from build123d import *

# Parameters (mm, degrees)
PAD_DEPTH            = 60
SKETCH001_R          = 1.45
POCKET_DEPTH         = 59
SKETCH002_R          = 1.5
POCKET001_DEPTH      = 13.501
POCKET001_DEPTH_BACK = -73.501
SKETCH003_R          = 7.75
POCKET002_DEPTH      = 333.774629
POLARPATTERN_COUNT   = 4
CHAMFER_SIZE         = 2


with BuildPart() as part:
    # Sketch → Pad (new body)
    with BuildSketch(Plane.XY):
        with BuildLine():
            Line((-39.5, 43.5), (39.5, 43.5))
            ThreePointArc((43.5, 39.5), (42.328427, 42.328427), (39.5, 43.5))
            Line((43.5, 39.5), (43.5, -39.5))
            ThreePointArc((39.5, -43.5), (42.328427, -42.328427), (43.5, -39.5))
            Line((39.5, -43.5), (-39.5, -43.5))
            ThreePointArc((-43.5, -39.5), (-42.328427, -42.328427), (-39.5, -43.5))
            Line((-43.5, -39.5), (-43.5, 39.5))
            ThreePointArc((-39.5, 43.5), (-42.328427, 42.328427), (-43.5, 39.5))
        make_face()
    extrude(amount=PAD_DEPTH)

    # Sketch001 (on Face10 of Pad) → Pocket (cut)
    with BuildSketch(Plane.XY.offset(60)):
        with Locations((-33, 33)):
            Circle(SKETCH001_R)
        with Locations((33, 33)):
            Circle(SKETCH001_R)
        with Locations((33, -33)):
            Circle(SKETCH001_R)
        with Locations((-33, -33)):
            Circle(SKETCH001_R)
        with BuildLine():
            Line((-30, 33), (-30, 41))
            Line((-30, 41), (30, 41))
            Line((30, 41), (30, 33))
            ThreePointArc((30, 33), (30.87868, 30.87868), (33, 30))
            Line((33, 30), (41, 30))
            Line((41, 30), (41, -30))
            Line((41, -30), (33, -30))
            ThreePointArc((33, -30), (30.87868, -30.87868), (30, -33))
            Line((30, -33), (30, -41))
            Line((30, -41), (-30, -41))
            Line((-30, -41), (-30, -33))
            ThreePointArc((-30, -33), (-30.87868, -30.87868), (-33, -30))
            Line((-33, -30), (-41, -30))
            Line((-41, -30), (-41, 30))
            Line((-41, 30), (-33, 30))
            ThreePointArc((-33, 30), (-30.87868, 30.87868), (-30, 33))
        make_face()
    extrude(amount=-POCKET_DEPTH, mode=Mode.SUBTRACT)

    # Sketch002 (on Face26 of Pocket) → Pocket001 (cut, two sides)
    with BuildSketch(Plane.XZ.offset(-30)) as pocket001_sk:
        with Locations((-37, 55)):
            Circle(SKETCH002_R)
        with Locations((37, 55)):
            Circle(SKETCH002_R)
        with Locations((-37, 6)):
            Circle(SKETCH002_R)
        with Locations((37, 6)):
            Circle(SKETCH002_R)
    extrude(amount=-POCKET001_DEPTH, mode=Mode.SUBTRACT)
    extrude(pocket001_sk.sketch, amount=-POCKET001_DEPTH_BACK, mode=Mode.SUBTRACT)

    # Sketch003 → Pocket002 (cut, through all)
    with BuildSketch(Plane.XY):
        with Locations((20, 20)):
            Circle(SKETCH003_R)
    pocket002 = extrude(amount=POCKET002_DEPTH, mode=Mode.SUBTRACT)

    # PolarPattern: Pocket002 ×4 about axis
    polarpattern_axis = Axis((0, 0, 0), (0, 0, 1))
    for i in range(1, POLARPATTERN_COUNT):
        add(pocket002.rotate(polarpattern_axis, i * 360 / POLARPATTERN_COUNT), mode=Mode.SUBTRACT)

    # Chamfer
    chamfer_edges = [part.edges().sort_by_distance(p)[0] for p in [
        (-37, 30, 1),
        (0, 41, 1),
        (30, 37, 1),
        (-41, 0, 1),
        (-30, -37, 1),
        (0, -41, 1),
        (41, 0, 1),
        (37, -30, 1),
    ]]
    chamfer(chamfer_edges, length=CHAMFER_SIZE)


solid = part.part
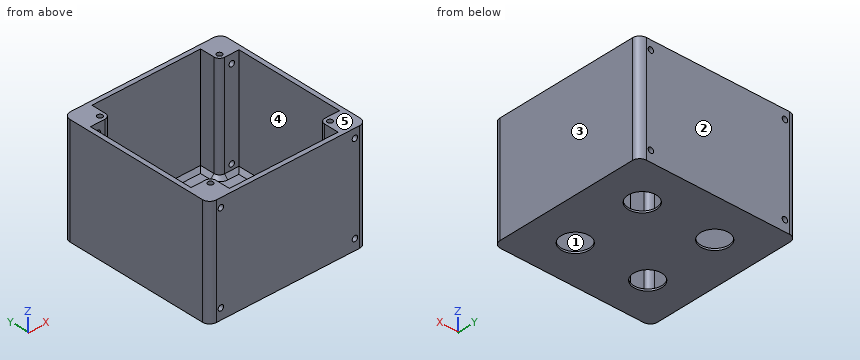
Part model, mm, in its own coordinate system. Face numbers are marked on the shaded views. A direction names the side the tool comes from. Give positions to 0.01 mm unless a question says otherwise; leave off trailing zeros. Write each loop counter-clockwise with the first axis right and the second up, starting at its lowest first coordinate (ties: lowest second). Pieces come first, ordered by that corner, then holes.
1) Probe L1, parallel to Z at x = 37, y = 37; L2, parallel to X at y = -37, z = 55; L3, parallel to Y at x = 20, z = 0.65. List the from-to ranges inside material, lowest first.
Resolved:
L1: z = 0 to 4.5, 7.5 to 53.5, 56.5 to 60
L2: x = -43.5 to -38.5, -35.5 to -30, 30 to 35.5, 38.5 to 43.5
L3: y = -43.5 to -27.75, -12.25 to 12.25, 27.75 to 43.5
2) Which spindle directions (+Z, -Z, +X, -X, +Y, -Y) get a long thin tool onto all of the face, cutting with end or side? Do the marked faces 4 and 5. Say none if no direction does.
Resolved:
face 4: +Z
face 5: +Z, +X, -X, +Y, -Y
3) Two-plate mould, pull along Y, no slides. Class the marked faces 1, 2 and 3: released by +Y, released by -Y, zero draft, split by the parting line, or undercut.
Resolved:
face 1: undercut
face 2: released by +Y
face 3: zero draft
4) Cut at C-C on z = 48. Write the cut outline in (x, y), then the cut area to 3 significant figures.
Resolved:
outline: (-43.5, -39.5) arc R4 ccw to (-39.5, -43.5) - (39.5, -43.5) arc R4 ccw to (43.5, -39.5) - (43.5, 39.5) arc R4 ccw to (39.5, 43.5) - (-39.5, 43.5) arc R4 ccw to (-43.5, 39.5) - close; hole (-41, -30) - (-33, -30) arc R3 cw to (-30, -33) - (-30, -41) - (30, -41) - (30, -33) arc R3 cw to (33, -30) - (41, -30) - (41, 30) - (33, 30) arc R3 cw to (30, 33) - (30, 41) - (-30, 41) - (-30, 33) arc R3 cw to (-33, 30) - (-41, 30) - close; hole circle Ø2.9 at (-33, -33); hole circle Ø2.9 at (-33, 33); hole circle Ø2.9 at (33, -33); hole circle Ø2.9 at (33, 33)
area: 1,280 mm2
5) Cut at A-A on x = -20. Write the cut outline in (y, z), then the cut area to 3 significant figures.
Resolved:
outline: (-43.5, 0) - (-27.75, 0) - (-27.75, 1) - (-39, 1) - (-41, 3) - (-41, 60) - (-43.5, 60) - close; (-12.25, 0) - (12.25, 0) - (12.25, 1) - (-12.25, 1) - close; (27.75, 0) - (43.5, 0) - (43.5, 60) - (41, 60) - (41, 3) - (39, 1) - (27.75, 1) - close
area: 355 mm2
6) Cut at D-D on y = -36.5. Write the cut outline in (x, z).
Resolved:
outline: (-43.5, 0) - (43.5, 0) - (43.5, 60) - (30, 60) - (30, 3) - (28, 1) - (-28, 1) - (-30, 3) - (-30, 60) - (-43.5, 60) - close; hole circle Ø3 at (-37, 6); hole circle Ø3 at (-37, 55); hole circle Ø3 at (37, 6); hole circle Ø3 at (37, 55)
7) Pin check, flat tips, straight feed: pin 1 (4 mm diameter, centred on x = 30.5, y = -21, fed in from +Z); pin 2 (1.8 mm diameter, centred on x = -37, z = 6, fed in from -Y). Stop position of each tip, or through.
Resolved:
pin 1: stops at z = 1
pin 2: passes through
